Read the model definition and answer for the solid it produces. Units are mm, in the model's axes. A direction names the side the tool comes from. Coordinates: 2 decimals unless noted, no trailing zeros. Write each loop counter-clockwise with the first axis right and the second up, starting at its lowest first coordinate (ties: lowest second). Pieces come first, ordered by that corner, then holes. Notation, with made-up numbers: (-39, 70) -> (17, 70) arc R20 cw to (17, 76) -> close; hole circle Ø8 at (2.25, 12.25). An arc over 180 degrees is marked (long way). Return JSON: item names as keys, results as strings.
from build123d import *

# Parameters (mm, degrees)
BOSS_EXTRUDE1_DEPTH = 150
SKETCH2_R           = 10
CUT_EXTRUDE1_DEPTH  = 150
SKETCH3_R           = 5
CUT_EXTRUDE2_DEPTH  = 273.07833604


with BuildPart() as part:
    # Sketch1 → Boss-Extrude1 (new body)
    with BuildSketch(Plane(origin=(0, 0, 0), x_dir=(0, 0, -1), z_dir=(1, 0, 0))):
        Polygon((7.362101983, -50), (7.362101983, 150), (107.362101983, 150), (107.362101983, 120), (37.362101983, 120), (37.362101983, -50), align=None)
    extrude(amount=BOSS_EXTRUDE1_DEPTH)

    # Sketch2 → Cut-Extrude1 (cut)
    with BuildSketch(Plane.XY.offset(-7.362101983)):
        with Locations((37.5, -25)):
            Circle(SKETCH2_R)
        with Locations((37.5, 15)):
            Circle(SKETCH2_R)
        with Locations((112.5, -25)):
            Circle(SKETCH2_R)
        with Locations((112.5, 15)):
            Circle(SKETCH2_R)
    extrude(amount=-CUT_EXTRUDE1_DEPTH, mode=Mode.SUBTRACT)

    # Sketch3 → Cut-Extrude2 (cut, through all)
    with BuildSketch(Plane(origin=(0, 150, 0), x_dir=(1, 0, 0), z_dir=(0, 1, 0))):
        with Locations(Location((15, 87.362101983, 0), (0, 0, 270))):
            Circle(SKETCH3_R)
        with Locations(Location((15, 47.362101983, 0), (0, 0, 270))):
            Circle(SKETCH3_R)
        with Locations(Location((135, 47.362101983, 0), (0, 0, 270))):
            Circle(SKETCH3_R)
        with Locations(Location((135, 87.362101983, 0), (0, 0, 270))):
            Circle(SKETCH3_R)
    extrude(amount=-CUT_EXTRUDE2_DEPTH, mode=Mode.SUBTRACT)


solid = part.part
1. Consider L1, parallel to Y at x = 37.5, z = -18; L2, parallel to Y at x = 118, z = -36; L3, parallel to Y at x = 45, z = -40. Determine where each line is inside the solid, lowest interval first.
Taken from the geometry:
{"L1": "y = -50 to -35, -15 to 5, 25 to 150", "L2": "y = -50 to -33.35, -16.65 to 6.65, 23.35 to 150", "L3": "y = 120 to 150"}
2. Flat-ended cylindrical pins translate along their axes: pin 1 Ø12 at (x, y) = (112.5, 15) entering from -Z; pin 2 Ø1 at (x, y) = (35, 95) entering from -Z. Find the tip coordinate at first contact, or state that the pin passes through.
Taken from the geometry:
{"pin 1": "passes through", "pin 2": "stops at z = -37.36"}
3. The part is cut by section B-B (z = -24.5). Determine the outline of the cut face in (x, y).
Taken from the geometry:
{"outline": "(0, -50) -> (150, -50) -> (150, 150) -> (0, 150) -> close; hole circle Ø20 at (37.5, -25); hole circle Ø20 at (37.5, 15); hole circle Ø20 at (112.5, -25); hole circle Ø20 at (112.5, 15)"}
4. The part is cut by section C-C (y = 15). Determine the outline of the cut face in (x, z).
Taken from the geometry:
{"outline": "(0, -37.36) -> (27.5, -37.36) -> (27.5, -7.36) -> (0, -7.36) -> close; (47.5, -37.36) -> (102.5, -37.36) -> (102.5, -7.36) -> (47.5, -7.36) -> close; (122.5, -37.36) -> (150, -37.36) -> (150, -7.36) -> (122.5, -7.36) -> close"}
5. For a pull along Y with two mould halves and no side action, classify faces 3 (the face through (74, -50, -23)), 4 (the face through (74, 49, -7.362)), 5 (the face through (36.198, 24.915, -22.152)) as +Y half, -Y half, draft (parallel to the pull), parting line (faces both ways), or undercut.
Taken from the geometry:
{"face 3": "-Y half", "face 4": "draft", "face 5": "undercut"}
6. The part is cut by section D-D (z = -48). Determine the outline of the cut face in (x, y).
Taken from the geometry:
{"outline": "(0, 120) -> (10.04, 120) -> (10.04, 150) -> (0, 150) -> close; (19.96, 120) -> (130.04, 120) -> (130.04, 150) -> (19.96, 150) -> close; (139.96, 120) -> (150, 120) -> (150, 150) -> (139.96, 150) -> close"}
7. The part is cut by section A-A (x = 37.5). Determine the outline of the cut face in (y, z), then the cut area to 3 significant figures.
Taken from the geometry:
{"outline": "(-50, -37.36) -> (-35, -37.36) -> (-35, -7.36) -> (-50, -7.36) -> close; (-15, -37.36) -> (5, -37.36) -> (5, -7.36) -> (-15, -7.36) -> close; (25, -37.36) -> (120, -37.36) -> (120, -107.36) -> (150, -107.36) -> (150, -7.36) -> (25, -7.36) -> close", "area": "6,900 mm2"}
8. A tool of negligible diameter and unlimited length cuts with its end or side. For faces 1 (the face through (74, 36, -37.362)), 2 (the face through (130.564, 135.21, -85.055)), from which of +Z, -Z, +X, -X, +Y, -Y can it reach the whole face along a straight path? Write none if from no direction.
Taken from the geometry:
{"face 1": "-Z, +X, -X, -Y", "face 2": "+Y, -Y"}
